Input: part model. Units: mm. Frame: model coordinates. A direction names the side the tool comes from. Coordinates: 2 decimals unless noted, no trailing zeros. Write each loop counter-clockwise with the first axis right and the second up, starting at its lowest first coordinate (ties: lowest second). Pieces come first, ordered by that corner, then holes. Notation, with made-up numbers: M -8.5,80.5 L 16.5,80.5 A16 ccw 16.5,96.5 Z; hole C 53.25,-2 d10. An arc over 180 degrees is marked long. Use CSV: the item, a comma, the result in double quotes.
```python
from build123d import *

# Parameters (mm, degrees)
BOSS_EXTRU_1_DEPTH      = 12.7
ESQUISSE3_W             = 0.8
ESQUISSE3_H             = 1.27
ENL_V_MAT_EXTRU_1_DEPTH = 8.9
ESQUISSE4_W             = 2.4
ESQUISSE4_H             = 0.5
ENL_V_MAT_EXTRU_2_DEPTH = 13.7
ESQUISSE2_W             = 0.6
ESQUISSE2_H             = 0.6
BOSS_EXTRU_2_DEPTH      = 3.5
BOSS_EXTRU_2_DEPTH_BACK = 9
BOSS_EXTRU_3_DEPTH      = 10.16
CHANFREIN4_SIZE         = 0.15
CHANFREIN5_SIZE         = 0.4


with BuildPart() as part:
    # Esquisse1 → Boss.-Extru.1 (new body)
    with BuildSketch(Plane.XY):
        Polygon((0, 11.4), (0, 0), (5, 0), (5, 11.4), (4.2, 11.4), (4.2, 2.5), (0.8, 2.5), (0.8, 11.4), align=None)
    extrude(amount=BOSS_EXTRU_1_DEPTH)

    # Esquisse3 → Enlèv. mat.-Extru.1 (cut)
    with BuildSketch(Plane(origin=(0, 11.4, 0), x_dir=(1, 0, 0), z_dir=(0, 1, 0))):
        with Locations((0.4, -0.635)):
            Rectangle(ESQUISSE3_W, ESQUISSE3_H)
        with Locations((0.4, -12.065)):
            Rectangle(ESQUISSE3_W, ESQUISSE3_H)
    extrude(amount=-ENL_V_MAT_EXTRU_1_DEPTH, mode=Mode.SUBTRACT)

    # Esquisse4 → Enlèv. mat.-Extru.2 (cut, through all)
    with BuildSketch(Plane.XY.offset(12.7)):
        with Locations((2.5, 0.25)):
            Rectangle(ESQUISSE4_W, ESQUISSE4_H)
    extrude(amount=-ENL_V_MAT_EXTRU_2_DEPTH, mode=Mode.SUBTRACT)

    # Esquisse2 → Boss.-Extru.2 (add, two sides)
    with BuildSketch(Plane.XZ.offset(-0.5)) as boss_extru_2_sk:
        with Locations((2.5, 11.43)):
            Rectangle(ESQUISSE2_W, ESQUISSE2_H)
        with Locations((2.5, 1.27)):
            Rectangle(ESQUISSE2_W, ESQUISSE2_H)
        with Locations((2.5, 8.89)):
            Rectangle(ESQUISSE2_W, ESQUISSE2_H)
        with Locations((2.5, 6.35)):
            Rectangle(ESQUISSE2_W, ESQUISSE2_H)
        with Locations((2.5, 3.81)):
            Rectangle(ESQUISSE2_W, ESQUISSE2_H)
    extrude(amount=BOSS_EXTRU_2_DEPTH)
    extrude(boss_extru_2_sk.sketch, amount=-BOSS_EXTRU_2_DEPTH_BACK)

    # Esquisse5 → Boss.-Extru.3 (add)
    with BuildSketch(Plane.XY.offset(11.43)):
        Polygon((0.8, 9.5), (1.2, 8.5), (0.8, 8.5), align=None)
    extrude(amount=-BOSS_EXTRU_3_DEPTH)

    # Chanfrein4
    chanfrein4_edges = [part.edges().sort_by_distance(p)[0] for p in [
        (2.8, 9.5, 8.89),
        (2.5, 9.5, 8.59),
        (2.2, 9.5, 8.89),
        (2.5, 9.5, 9.19),
        (2.8, -3, 8.89),
        (2.5, -3, 9.19),
        (2.2, -3, 8.89),
        (2.5, -3, 8.59),
        (2.8, 9.5, 6.35),
        (2.5, 9.5, 6.05),
        (2.2, 9.5, 6.35),
        (2.5, 9.5, 6.65),
        (2.8, -3, 6.35),
        (2.5, -3, 6.65),
        (2.2, -3, 6.35),
        (2.5, -3, 6.05),
        (2.8, 9.5, 3.81),
        (2.5, 9.5, 3.51),
        (2.2, 9.5, 3.81),
        (2.5, 9.5, 4.11),
        (2.8, -3, 3.81),
        (2.5, -3, 4.11),
        (2.2, -3, 3.81),
        (2.5, -3, 3.51),
        (2.8, 9.5, 11.43),
        (2.5, 9.5, 11.13),
        (2.2, 9.5, 11.43),
        (2.5, 9.5, 11.73),
        (2.8, -3, 11.43),
        (2.5, -3, 11.73),
        (2.2, -3, 11.43),
        (2.5, -3, 11.13),
        (2.8, 9.5, 1.27),
        (2.5, 9.5, 0.97),
        (2.2, 9.5, 1.27),
        (2.5, 9.5, 1.57),
        (2.8, -3, 1.27),
        (2.5, -3, 1.57),
        (2.2, -3, 1.27),
        (2.5, -3, 0.97),
    ]]
    chamfer(chanfrein4_edges, length=CHANFREIN4_SIZE)

    # Chanfrein5
    chanfrein5_edges = [part.edges().sort_by_distance(p)[0] for p in [
        (4.2, 11.4, 6.35),
        (0.8, 11.4, 6.35),
    ]]
    chamfer(chanfrein5_edges, length=CHANFREIN5_SIZE)


solid = part.part
```
1. Mould query, pull axis Y, two halves, no side actions, for faces 1 (the flat face through (1, 9, 6)), 2 (the flat face through (4, 0, 6)), 3 (the flat face through (0.8, 5, 6)), 4 (the flat face through (4.2, 7, 6)). Classes: pulls with the +Y half, pulls with the -Y half, needs draft (parallel to the pull), parting line crosses it, or undercut.
Resolved:
face 1,"pulls with the +Y half"
face 2,"pulls with the -Y half"
face 3,"undercut"
face 4,"needs draft"
2. Access query for faces 5 (the flat face through (0.5, 7, 11.43)), 6 (the flat face through (3, 2, 12.7)), 7 (the flat face through (0.5, 7, 1.27)), 8 (the flat face through (0.8, 10, 6)), 9 (the flat face through (1, 0, 6)). Directions: +Z, -Z, +X, -X, +Y, -Y. A direction counts if a zero-diameter tool reaches every point of the face in a straight line with its end or side. Return the directions, or none.
Resolved:
face 5,"+Z, -X, +Y"
face 6,"+Z, +X, -X, +Y, -Y"
face 7,"-Z, -X, +Y"
face 8,"+Z, -Z, +Y"
face 9,"+Z, -Z, -X, -Y"
3. Section A-A (y = -0.25). Return loops of the section in (x, z), then the cut area to 3 significant figures.
Resolved:
outline,"M 2.2,0.97 L 2.8,0.97 L 2.8,1.57 L 2.2,1.57 Z; M 2.2,3.51 L 2.8,3.51 L 2.8,4.11 L 2.2,4.11 Z; M 2.2,6.05 L 2.8,6.05 L 2.8,6.65 L 2.2,6.65 Z; M 2.2,8.59 L 2.8,8.59 L 2.8,9.19 L 2.2,9.19 Z; M 2.2,11.13 L 2.8,11.13 L 2.8,11.73 L 2.2,11.73 Z"
area,"1.80 mm^2"
4. Section D-D (x = 1.5). Return loops of the section in (y, z), then the cut area to 3 significant figures.
Resolved:
outline,"M 0.5,0 L 2.5,0 L 2.5,12.7 L 0.5,12.7 Z"
area,"25.4 mm^2"
5. Section C-C (y = 3). Return loops of the section in (x, z).
Resolved:
outline,"M 0,1.27 L 0.8,1.27 L 0.8,11.43 L 0,11.43 Z; M 2.2,0.97 L 2.8,0.97 L 2.8,1.57 L 2.2,1.57 Z; M 2.2,3.51 L 2.8,3.51 L 2.8,4.11 L 2.2,4.11 Z; M 2.2,6.05 L 2.8,6.05 L 2.8,6.65 L 2.2,6.65 Z; M 2.2,8.59 L 2.8,8.59 L 2.8,9.19 L 2.2,9.19 Z; M 2.2,11.13 L 2.8,11.13 L 2.8,11.73 L 2.2,11.73 Z; M 4.2,0 L 5,0 L 5,12.7 L 4.2,12.7 Z"
6. Material intervals for line 1 (X direction, y = 4.75, z = 4.75); line 2 (X direction, y = 4.75, z = 6.25); line 3 (Y direction, x = 2.7, z = 9.5), sorted ascending. Write a range as [from, to].
Resolved:
line 1,"x = [0, 0.8], [4.2, 5]"
line 2,"x = [0, 0.8], [2.2, 2.8], [4.2, 5]"
line 3,"y = [0.5, 2.5]"
7. Contact query for flat-ended pins moving along their axis: pin 1 Ø0.5 at (y, z) = (-1, 11.5) entering from -X; pin 2 Ø0.5 at (x, y) = (2.5, -0.5) entering from +Z; pin 3 Ø0.7 at (x, y) = (2.5, -2) entering from -Z. Output: stop coordinate, or through.
Resolved:
pin 1,"stops at x = 2.2"
pin 2,"stops at z = 11.73"
pin 3,"stops at z = 0.97"
8. Section B-B (z = 12.25). Return loops of the section in (x, y).
Resolved:
outline,"M 0,0 L 1.3,0 L 1.3,0.5 L 3.7,0.5 L 3.7,0 L 5,0 L 5,11.4 L 4.6,11.4 L 4.2,11 L 4.2,2.5 L 0,2.5 Z"
